from build123d import *

# Parameters (mm, degrees)
SKETCH1_W                   = 15
SKETCH1_H                   = 15
BOSS_EXTRUDE1_DEPTH         = 3.175
SKETCH2_W                   = 2.75
SKETCH2_H                   = 2.5
SKETCH2_H_2                 = 4
SKETCH2_W_2                 = 1.125
SKETCH2_H_3                 = 7.5
CUT_EXTRUDE1_DEPTH          = 141.379634965
CIRPATTERN1_COUNT           = 4
F_3_0_3_DIAMETER_HOLE1_D    = 3
F_1_2_CLEARANCE_HOLE1_D     = 13.89126
F_1_2_CLEARANCE_HOLE1_DEPTH = 6.35


with BuildPart() as part:
    # Sketch1 → Boss-Extrude1 (new, symmetric)
    with BuildSketch(Plane(origin=(0, 0, 0), x_dir=(1, 0, 0), z_dir=(0, 1, 0))):
        with BuildLine():
            Line((-83.903460262, -7.5), (-98.95418457, -7.5))
            ThreePointArc((-98.95418457, -7.5), (-70.171862751, -70.171862751), (-7.5, -98.95418457))
            Line((-7.5, -98.95418457), (-7.5, -83.903460262))
            ThreePointArc((-7.5, -83.903460262), (-59.565261034, -59.565261034), (-83.903460262, -7.5))
        make_face()
        with BuildLine():
            ThreePointArc((-98.95418457, 7.5), (-99.238, 0), (-98.95418457, -7.5))
            Line((-98.95418457, -7.5), (-83.903460262, -7.5))
            ThreePointArc((-83.903460262, -7.5), (-84.238, 0), (-83.903460262, 7.5))
            Line((-83.903460262, 7.5), (-98.95418457, 7.5))
        make_face()
        with BuildLine():
            Line((83.903460262, -7.5), (98.95418457, -7.5))
            ThreePointArc((98.95418457, -7.5), (99.167020759, -3.752684079), (99.238, 0))
            ThreePointArc((99.238, 0), (99.167020759, 3.752684079), (98.95418457, 7.5))
            Line((98.95418457, 7.5), (83.903460262, 7.5))
            ThreePointArc((83.903460262, 7.5), (84.154323506, 3.753728707), (84.238, 0))
            ThreePointArc((84.238, 0), (84.154323506, -3.753728707), (83.903460262, -7.5))
        make_face()
        with BuildLine():
            ThreePointArc((-7.5, 98.95418457), (-70.171862751, 70.171862751), (-98.95418457, 7.5))
            Line((-98.95418457, 7.5), (-83.903460262, 7.5))
            ThreePointArc((-83.903460262, 7.5), (-59.565261034, 59.565261034), (-7.5, 83.903460262))
            Line((-7.5, 83.903460262), (-7.5, 98.95418457))
        make_face()
        with BuildLine():
            Line((-7.5, -83.903460262), (-7.5, -98.95418457))
            ThreePointArc((-7.5, -98.95418457), (0, -99.238), (7.5, -98.95418457))
            Line((7.5, -98.95418457), (7.5, -83.903460262))
            ThreePointArc((7.5, -83.903460262), (0, -84.238), (-7.5, -83.903460262))
        make_face()
        with BuildLine():
            ThreePointArc((7.5, 98.95418457), (0, 99.238), (-7.5, 98.95418457))
            Line((-7.5, 98.95418457), (-7.5, 83.903460262))
            ThreePointArc((-7.5, 83.903460262), (0, 84.238), (7.5, 83.903460262))
            Line((7.5, 83.903460262), (7.5, 98.95418457))
        make_face()
        with BuildLine():
            ThreePointArc((98.95418457, 7.5), (70.171862751, 70.171862751), (7.5, 98.95418457))
            Line((7.5, 98.95418457), (7.5, 83.903460262))
            ThreePointArc((7.5, 83.903460262), (59.565261034, 59.565261034), (83.903460262, 7.5))
            Line((83.903460262, 7.5), (98.95418457, 7.5))
        make_face()
        with BuildLine():
            Line((7.5, -83.903460262), (7.5, -98.95418457))
            ThreePointArc((7.5, -98.95418457), (70.171862751, -70.171862751), (98.95418457, -7.5))
            Line((98.95418457, -7.5), (83.903460262, -7.5))
            ThreePointArc((83.903460262, -7.5), (59.565261034, -59.565261034), (7.5, -83.903460262))
        make_face()
        with BuildLine():
            Line((7.5, -7.5), (-7.5, -7.5))
            Line((-7.5, -7.5), (-7.5, -83.903460262))
            ThreePointArc((-7.5, -83.903460262), (0, -84.238), (7.5, -83.903460262))
            Line((7.5, -83.903460262), (7.5, -7.5))
        make_face()
        with BuildLine():
            ThreePointArc((-83.903460262, 7.5), (-84.238, 0), (-83.903460262, -7.5))
            Line((-83.903460262, -7.5), (-7.5, -7.5))
            Line((-7.5, -7.5), (-7.5, 7.5))
            Line((-7.5, 7.5), (-83.903460262, 7.5))
        make_face()
        with BuildLine():
            Line((-7.5, 83.903460262), (-7.5, 7.5))
            Line((-7.5, 7.5), (7.5, 7.5))
            Line((7.5, 7.5), (7.5, 83.903460262))
            ThreePointArc((7.5, 83.903460262), (0, 84.238), (-7.5, 83.903460262))
        make_face()
        with BuildLine():
            Line((7.5, 7.5), (7.5, -7.5))
            Line((7.5, -7.5), (83.903460262, -7.5))
            ThreePointArc((83.903460262, -7.5), (84.154323506, -3.753728707), (84.238, 0))
            ThreePointArc((84.238, 0), (84.154323506, 3.753728707), (83.903460262, 7.5))
            Line((83.903460262, 7.5), (7.5, 7.5))
        make_face()
        Rectangle(SKETCH1_W, SKETCH1_H)
    extrude(amount=BOSS_EXTRUDE1_DEPTH, both=True)

    # Sketch2 → Cut-Extrude1 (cut, symmetric)
    with BuildSketch(Plane(origin=(0, 0, 0), x_dir=(1, 0, 0), z_dir=(0, 1, 0))):
        with Locations((0, 86.488)):
            Rectangle(SKETCH2_W, SKETCH2_H)
        with Locations((0, 89.738)):
            Rectangle(SKETCH2_W, SKETCH2_H_2)
        with Locations((1.9375, 89.738)):
            Rectangle(SKETCH2_W_2, SKETCH2_H_2)
        with Locations((0, 95.488)):
            Rectangle(SKETCH2_W, SKETCH2_H_3)
        with Locations((-1.9375, 89.738)):
            Rectangle(SKETCH2_W_2, SKETCH2_H_2)
    cut_extrude1 = extrude(amount=CUT_EXTRUDE1_DEPTH, both=True, mode=Mode.SUBTRACT)

    # CirPattern1: Cut-Extrude1 ×4 about axis
    cirpattern1_axis = Axis((0, 0, 0), (0, 1, 0))
    for i in range(1, CIRPATTERN1_COUNT):
        add(cut_extrude1.rotate(cirpattern1_axis, i * 360 / CIRPATTERN1_COUNT), mode=Mode.SUBTRACT)

    # Ø3.0 (3) Diameter Hole1 (through all)
    with Locations(Plane(origin=(0, 3.175, 0), x_dir=(1, 0, 0), z_dir=(0, 1, 0))):
        with Locations((-64.868561892, -64.868561892), (0, 0), (-64.868561892, 64.868561892), (64.868561892, 64.868561892), (64.868561892, -64.868561892)):
            Hole(F_3_0_3_DIAMETER_HOLE1_D / 2)

    # 1/2 Clearance Hole1
    with Locations(Plane(origin=(0, 3.175, 0), x_dir=(1, 0, 0), z_dir=(0, 1, 0))):
        with Locations((0, 0)):
            Hole(F_1_2_CLEARANCE_HOLE1_D / 2, depth=F_1_2_CLEARANCE_HOLE1_DEPTH)


solid = part.part
Model file for the job. Use its own axes, mm. A direction names the side the tool comes from. Give positions to 0.01 mm unless a question says otherwise; leave off trailing zeros. Order: outer loops, then holes, each group sorted by start corner. A loop starts at its lowest first (then second) coordinate and runs counter-clockwise, first axis right, second up. Notation, with made-up numbers: M -14,-21 L 28,-21 A22 ccw 28,-15 Z; hole C 69.5,63.5 d5. An arc over 180 degrees is marked long. Write item = value, one per line.
Q1. Flat gauge pins, fed straight in: pin 1 (0.6 mm diameter, centred on y = 1.5, z = 2, fed in from +X); pin 2 (0.9 mm diameter, centred on y = -0.5, z = 2, fed in from -X); pin 3 (1.2 mm diameter, centred on x = 89, y = -1.5, fed in from +Z). Where does each tip first touch, or does it go through?
Derived:
pin_1 = 99.22
pin_2 = -99.23
pin_3 = 45.1
Q2. Cut at C-C, the plane y = -1. Count the separate pieces of the cut face and the enclosed holes in it, then the cut area to 3 significant figures.
Derived:
separate_pieces = 1
enclosed_holes = 9
area = 13,100 mm2
Q3. Drill centre lines: line 1 (Z direction, x = -36, y = 0); line 2 (X direction, y = -0.75, z = 29.5); line 3 (X direction, y = 0.5, z = -41). Where is each one in solid material? Low to high. Write a range as [from, to].
Derived:
line_1 = [-92.48, -76.16], [-7.5, 7.5], [76.16, 92.48]
line_2 = [-94.75, -78.9], [-7.5, 7.5], [78.9, 94.75]
line_3 = [-90.37, -73.59], [-7.5, 7.5], [73.59, 90.37]
Q4. Cut at B-B, the plane x = 33. List the corners of the cut face in (y, z) (1 decimal), then the cut area to 3 significant figures.
Derived:
outline = M -3.2,-93.6 L 3.2,-93.6 L 3.2,-77.5 L -3.2,-77.5 Z; M -3.2,-7.5 L 3.2,-7.5 L 3.2,7.5 L -3.2,7.5 Z; M -3.2,77.5 L 3.2,77.5 L 3.2,93.6 L -3.2,93.6 Z
area = 300 mm2
Q5. Two-plate mould, pull along Z, no slides. Class faces 5 (the flat face through (-45, 0, -7.5)), 6 (the cylindrical face through (-60.143, 0.044, -58.982)), 7 (the flat face through (1.375, 0, 96)): pulls with the +Z half, pulls with the -Z half, needs draft (parallel to the pull), parting line crosses it, or undercut.
Derived:
face_5 = undercut
face_6 = undercut
face_7 = needs draft
Q6. Tool access for faces 1 (the cylindrical face through (58.982, 0.044, -60.143)), 2 (the flat face through (1.375, 0, -95)), 3 (the flat face through (-96, 0, 1.375)), 4 (the flat face through (95, 0, 1.375)): list every direction of +Z, -Z, +X, -X, +Y, -Y with a clear straight run to the whole face (end or side of a thin tool).
Derived:
face_1 = +Y, -Y
face_2 = -Z, +Y, -Y
face_3 = -X, +Y, -Y
face_4 = +X, +Y, -Y
Q7. Cut at A-A, the plane z = 20. List the corners of the cut face in (x, y) (3 decimals).
Derived:
outline = M -97.202,-3.175 L -81.829,-3.175 L -81.829,3.175 L -97.202,3.175 Z; M -7.5,-3.175 L 7.5,-3.175 L 7.5,3.175 L -7.5,3.175 Z; M 81.829,-3.175 L 97.202,-3.175 L 97.202,3.175 L 81.829,3.175 Z
